Geometry check sheet. Reference: drawing and pictorial views, mm from the part's lowest x, y, z. Round coordinates to 2 decimals unless told otherwise and drop trailing zeros. Use one line per item in the form item = value. Start each with the question number.
(1) Material ranges on probe 1 along X at (y, z) = (1, 25.5) (1 decimal); probe 2 along X at (y, z) = (4.75, 63.5) (1 decimal); probe 3 along Z at (x, y) = (270.5, 1.5) (1 decimal), recorded low to high. Write a range as [from, to].
(2) Go/stop test with a flat-tipped pin: pin 1 (1.9 mm diameter, centred on x = 6.35, z = 12.7, fed in from +Y). Record where the tip stops, or that it passes through.
(3) Sectioned sample at A-A (z = 35). State how many separate pieces and enclosed holes the cut face has, and give its area (3 significant figures).
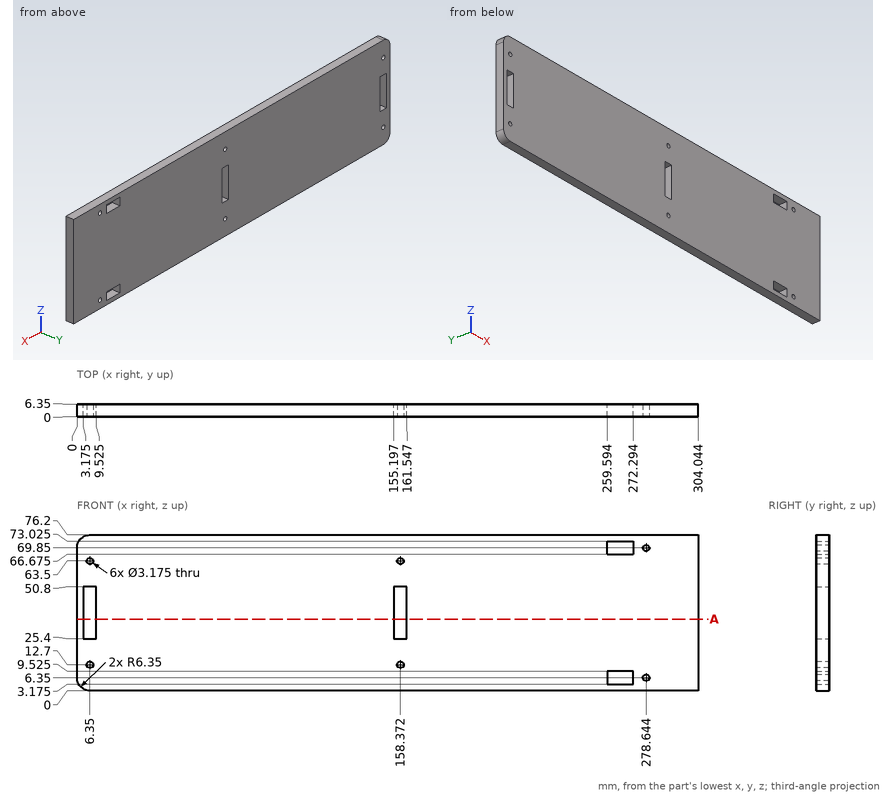
Checks:
q1.probe_1 = [0, 3.2], [9.5, 155.2], [161.5, 304]
q1.probe_2 = [0, 4.8], [7.9, 156.8], [160, 304]
q1.probe_3 = [0, 3.2], [9.5, 66.7], [73, 76.2]
q2.pin_1 = through
q3.separate_pieces = 3
q3.enclosed_holes = 0
q3.area = 1,850 mm2
